```python
from build123d import *

# Parameters (mm, degrees)
SKETCH1_R           = 1.25
BOSS_EXTRUDE1_DEPTH = 3
SKETCH2_R           = 5
BOSS_EXTRUDE2_DEPTH = 5
FILLET1_R           = 2.5
SKETCH3_W           = 5
SKETCH3_H           = 29
SKETCH3_W_2         = 9.2
SKETCH3_H_2         = 13.8
SKETCH3_W_3         = 25
SKETCH3_W_4         = 50
SKETCH3_R           = 1.25
CUT_EXTRUDE1_DEPTH  = 9
FILLET2_R           = 1.5


with BuildPart() as part:
    # Sketch1 → Boss-Extrude1 (new body)
    with BuildSketch(Plane(origin=(0, 0, 0), x_dir=(1, 0, 0), z_dir=(0, 1, 0))):
        Polygon((-20.5, -38), (20.5, -38), (20.5, -32), (120.5, -32), (120.5, 32), (20.5, 32), (20.5, 38), (-20.5, 38), (-20.5, 24.5), (-40, 24.5), (-40, -24.5), (-20.5, -24.5), align=None)
        with Locations((-35.5, 20)):
            Circle(SKETCH1_R, mode=Mode.SUBTRACT)
        with Locations((-35.5, -20)):
            Circle(SKETCH1_R, mode=Mode.SUBTRACT)
    extrude(amount=BOSS_EXTRUDE1_DEPTH)

    # Sketch2 → Boss-Extrude2 (add)
    with BuildSketch(Plane(origin=(0, 3, 0), x_dir=(1, 0, 0), z_dir=(0, 1, 0))):
        with Locations((-9.925, 0)):
            Circle(SKETCH2_R)
        with Locations((9.925, 0)):
            Circle(SKETCH2_R)
    extrude(amount=BOSS_EXTRUDE2_DEPTH)

    # Fillet1
    fillet1_edges = [part.edges().sort_by_distance(p)[0] for p in [
        (-14.925, 3, 0),
        (4.925, 3, 0),
    ]]
    fillet(fillet1_edges, radius=FILLET1_R)

    # Sketch3 → Cut-Extrude1 (cut, through all)
    with BuildSketch(Plane(origin=(0, 0, 0), x_dir=(-1, 0, 0), z_dir=(0, -1, 0))):
        with Locations((-23, 0)):
            Rectangle(SKETCH3_W, SKETCH3_H)
        with BuildLine():
            Line((0.5, 9), (7.5, 9))
            ThreePointArc((7.5, 9), (10, 11.5), (7.5, 14))
            Line((7.5, 14), (0.5, 14))
            ThreePointArc((0.5, 14), (-2, 11.5), (0.5, 9))
        make_face()
        with BuildLine():
            Line((0.5, -14), (7.5, -14))
            ThreePointArc((7.5, -14), (10, -11.5), (7.5, -9))
            Line((7.5, -9), (0.5, -9))
            ThreePointArc((0.5, -9), (-2, -11.5), (0.5, -14))
        make_face()
        with Locations((30.25, 0)):
            Rectangle(SKETCH3_W_2, SKETCH3_H_2)
        with Locations((-108, 0)):
            Rectangle(SKETCH3_W_3, SKETCH3_H)
        with Locations((-60.5, 0)):
            Rectangle(SKETCH3_W_4, SKETCH3_H)
        with Locations((-30.5, -20)):
            Circle(SKETCH3_R)
        with Locations((-90.5, -20)):
            Circle(SKETCH3_R)
        with Locations((-30.5, 20)):
            Circle(SKETCH3_R)
        with Locations((-90.5, 20)):
            Circle(SKETCH3_R)
        with Locations((-7.25, 32.5)):
            Circle(SKETCH3_R)
        with Locations((15.25, 32.5)):
            Circle(SKETCH3_R)
        with Locations((-9.925, 0)):
            Circle(SKETCH3_R)
        with Locations((9.925, 0)):
            Circle(SKETCH3_R)
        with Locations((15.25, -32.5)):
            Circle(SKETCH3_R)
        with Locations((-7.25, -32.5)):
            Circle(SKETCH3_R)
    extrude(amount=-CUT_EXTRUDE1_DEPTH, mode=Mode.SUBTRACT)

    # Fillet2
    fillet2_edges = [part.edges().sort_by_distance(p)[0] for p in [
        (95.5, 1.5, -14.5),
        (95.5, 1.5, 14.5),
        (20.5, 1.5, 14.5),
        (25.5, 1.5, 14.5),
        (25.5, 1.5, -14.5),
        (20.5, 1.5, -14.5),
        (35.5, 1.5, -14.5),
        (35.5, 1.5, 14.5),
        (85.5, 1.5, 14.5),
        (85.5, 1.5, -14.5),
        (-20.5, 1.5, -38),
        (20.5, 1.5, -38),
        (20.5, 1.5, -32),
        (120.5, 1.5, -32),
        (120.5, 1.5, 32),
        (20.5, 1.5, 32),
        (20.5, 1.5, 38),
        (-20.5, 1.5, 38),
        (-20.5, 1.5, 24.5),
        (-40, 1.5, 24.5),
        (-40, 1.5, -24.5),
        (-20.5, 1.5, -24.5),
        (120.5, 1.5, -14.5),
        (120.5, 1.5, 14.5),
    ]]
    fillet(fillet2_edges, radius=FILLET2_R)


solid = part.part
```
Check sheet for the modelled part. Datum: model origin and axes. Units: mm. A direction names the side the tool comes from. Coordinates: 2 decimals unless noted, no trailing zeros. Loops run counter-clockwise (first coordinate to the right, second up) from the corner with the lowest first, then second, coordinate; pieces in that order, holes last.
1) Sectioned sample at B-B (z = -11.5). Record the boundary of the cut face in (x, y).
2) Access from +Z, -Z, +X, -X, +Y, -Y to the whole of each face (thin tool, end or side, straight path). Record for faces 5 (the face through (-14.92, 6.73, -0.22)), 6 (the face through (95.5, 1, 0)), 7 (the face through (2, 1.5, 11.4)), 8 (the face through (71, 1, -32)).
3) Release check for a two-part mould opening along X. For faces 1 (the face through (-20.5, 1, 31)), 2 (the face through (-4, 1, 14)), 3 (the face through (70, 1, 32)), 4 (the face through (-25.65, 1, 0)) record: released by +X, released by -X, zero draft, split by the parting line, or undercut.
4) Gauge pin test, flat ends, axial feed: pin 1 (3.5 mm diameter, centred on y = 2, z = -6.5, fed in from +X); pin 2 (1.5 mm diameter, centred on x = 59, y = 1.5, fed in from +Z); pin 3 (2 mm diameter, centred on x = 7.25, z = -32.5, fed in from +Y); pin 4 (0.9 mm diameter, centred on x = 106, y = 2, fed in from -Z). Record the tip position at first contact, or that the pin passes through.
5) Sectioned sample at C-C (y = 1.5). Count the separate pieces of the cut face and the enclosed holes in it, and give its area (3 significant figures).
6) Sectioned sample at A-A (x = 74). Record the boundary of the cut face in (y, z).
7) Sectioned sample at D-D (z = -27.5). Record the boundary of the cut face in (x, y), and give its area (3 significant figures).
8) Material ranges on probe 1 along Z at (x, y) = (7.25, 2.4); probe 2 along X at (y, z) = (1, -5); probe 3 along X at (y, z) = (0.5, 7.5), recorded low to high.
Check sheet entries:
1. outline: (-40, 0) - (-10, 0) - (-10, 3) - (-40, 3) - close; (2, 0) - (20.5, 0) - (20.5, 3) - (2, 3) - close; (25.5, 0) - (35.5, 0) - (35.5, 3) - (25.5, 3) - close; (85.5, 0) - (95.5, 0) - (95.5, 3) - (85.5, 3) - close
2. face 5: +Y
2. face 6: +X, +Y, -Y
2. face 7: +Y, -Y
2. face 8: -Z, +X, +Y, -Y
3. face 1: released by -X
3. face 2: undercut
3. face 3: zero draft
3. face 4: undercut
4. pin 1: stops at x = 95.5
4. pin 2: stops at z = 32
4. pin 3: passes through
4. pin 4: stops at z = -32
5. separate pieces: 1
5. enclosed holes: 17
5. area: 7,860 mm2
6. outline: (0, -32) - (3, -32) - (3, -14.5) - (0, -14.5) - close; (0, 14.5) - (3, 14.5) - (3, 32) - (0, 32) - close
7. outline: (-20.5, 0) - (120.5, 0) - (120.5, 3) - (-20.5, 3) - close
7. area: 423 mm2
8. probe 1: z = -38 to -33.75, -31.25 to 31.25, 33.75 to 38
8. probe 2: x = -40 to -34.85, -25.65 to 20.5, 25.5 to 35.5, 85.5 to 95.5
8. probe 3: x = -40 to 20.5, 25.5 to 35.5, 85.5 to 95.5
